Geometry: final body of the model. Coordinates: model frame, mm. Give positions to 0.01 mm unless a question says otherwise; leave off trailing zeros. Write each loop counter-clockwise with the first axis right and the second up, starting at its lowest first coordinate (ties: lowest second). Pieces come first, ordered by that corner, then holes.
Q1. Pin query (flat end, axial travel): pin 1 Ø1.9 at (x, z) = (20, -45) entering from -Y. Return the tip coordinate at first contact, or that it passes through.
Q2. Mould query, pull axis Z, two halves, no side actions, for faces 1 (the cylindrical face through (-19.26, 15.21, 46.42)), 2 (the cylindrical face through (18.73, 15.21, 45.97)), 3 (the flat face through (25, 15, -1)), 4 (the flat face through (0, 15, 50)). Classes: +Z half, -Z half, draft (parallel to the pull), parting line (faces both ways), or undercut.
Q3. Line query: line 1 (Z direction, x = 20, y = 20); line 2 (X direction, y = 7.5, z = 45). Output: solid intervals per line, ascending.
Q4. Section A-A (z = -45). Return the cut outline in (x, y), plus the area to 3 significant figures.
Q5. Section B-B (x = 20). Return the cut outline in (y, z).
Autodesk Inventor part; units mm, degrees
ref_plane "YZ Plane" through (0, 0, 0) normal (1, 0, 0) x (0, 1, 0)
ref_plane "XZ Plane" through (0, 0, 0) normal (0, 1, 0) x (-1, 0, 0)
ref_plane "XY Plane" through (0, 0, 0) normal (0, 0, 1) x (1, 0, 0)
sketch "Эскиз1" plane through (0, 0, 0) normal (0, 1, 0) x (-1, 0, 0)
  line L0 (-25, 50) -> (25, 50)
  line L1 (25, 50) -> (25, -50)
  line L2 (25, -50) -> (-25, -50)
  line L3 (-25, -50) -> (-25, 50)
  line L4 (-25, 50) -> (25, -50) construction
  line L5 (25, 50) -> (-25, -50) construction
  point P0 (0, 0)
  dimension "d0" = 50
  dimension "d1" = 100
extrude "Выдавливание1" add sketch "Эскиз1" along normal blind 30
sketch "Эскиз2" plane through (0, 30, 0) normal (0, 1, 0) x (1, 0, 0)
  line L0 (25, 50) -> (-25, 50)
  line L1 (-25, 50) -> (-25, -50)
  line L2 (-25, -50) -> (25, -50)
  line L3 (25, -50) -> (25, 50)
  circle A0 centre (20, 45) radius 1.6
  circle A1 centre (20, -45) radius 1.6
  circle A2 centre (-20, -45) radius 1.6
  arc A3 (-20, 52.5) -> (-25, 47.5) centre (-20, 45) ccw
  circle A4 centre (-20, 45) radius 1.6
  circle A5 centre (-20, 45) radius 5
  circle A6 centre (20, 45) radius 5
  circle A7 centre (20, -45) radius 5
  circle A8 centre (-20, -45) radius 5
  line L4 (-25, 50) -> (-25, -50)
  line L5 (-25, -50) -> (25, -50)
  line L6 (25, -50) -> (25, 50)
  line L7 (25, 50) -> (-25, 50)
  point P0 (0, 0)
  dimension "d5" = 3.2
  dimension "d6" = 3.2
  dimension "d7" = 3.2
  dimension "d8" = 3.2
  dimension "d11" = 10
  dimension "d12" = 10
  dimension "d13" = 10
  dimension "d14" = 10
extrude "Выдавливание2" cut sketch "Эскиз2" against normal blind 30 contours A0 | A1 | A2 | A4
sketch "Эскиз3" plane through (0, 0, 0) normal (0, -1, 0) x (1, 0, 0)
  line L0 (25, -50) -> (-25, -50)
  line L1 (0, -50) -> (0, 30)
  line L2 (0, 30) -> (25, 30)
  line L3 (25, 50) -> (25, -50)
  line L4 (-25, 50) -> (25, 50)
  line L5 (25, 50) -> (15, 50)
  line L6 (15, 50) -> (15, 30)
  circle A0 centre (-20, -45) radius 1.6
  circle A1 centre (20, 45) radius 1.6
  circle A2 centre (20, -45) radius 1.6
  circle A3 centre (-20, 45) radius 1.6
  line L7 (25, -50) -> (-25, -50)
  line L8 (25, 50) -> (25, -50)
  line L9 (-25, 50) -> (25, 50)
  line L10 (-25, -50) -> (-25, 50)
  point P0 (0, 0)
  dimension "d15" = 80
  dimension "d16" = 25
  dimension "d17" = 10
  dimension "d18" = 20
sketch "Эскиз4" plane through (-25, 0, -50) normal (-1, 0, 0) x (0, 0, 1)
  point P0 (50, 0)
properties part number "LPS_board"
Computed:
1. pin 1: passes through
2. face 1: undercut
2. face 2: undercut
2. face 3: draft
2. face 4: +Z half
3. line 1: z = -50 to -46.6, -43.4 to 43.4, 46.6 to 50
3. line 2: x = -25 to -21.6, -18.4 to 18.4, 21.6 to 25
4. outline: (-25, 0) - (-21.6, 0) - (-21.6, 30) - (-25, 30) - close; (-18.4, 0) - (18.4, 0) - (18.4, 30) - (-18.4, 30) - close; (21.6, 0) - (25, 0) - (25, 30) - (21.6, 30) - close
4. area: 1,310 mm2
5. outline: (0, -50) - (30, -50) - (30, -46.6) - (0, -46.6) - close; (0, -43.4) - (30, -43.4) - (30, 43.4) - (0, 43.4) - close; (0, 46.6) - (30, 46.6) - (30, 50) - (0, 50) - close
